For this review, take the finished solid that the model builds, in its own axes (mm). Round coordinates to 2 decimals unless told otherwise and drop trailing zeros. Write each loop counter-clockwise with the first axis right and the second up, starting at its lowest first coordinate (ties: lowest second). Pieces come first, ordered by that corner, then holes. Notation, with made-up numbers: (74.25, 36.25) - (106.25, 36.25) arc R24 ccw to (106.25, 51.25) - close; hole circle Ø4 at (9.25, -20). An arc over 180 degrees is marked (long way). Answer in a Markdown table with one row per item. Add a question column.
from build123d import *

# Parameters (mm, degrees)
SKETCH1_R           = 3.175
BOSS_EXTRUDE1_DEPTH = 3.175


with BuildPart() as part:
    # Sketch1 → Boss-Extrude1 (new body)
    with BuildSketch(Plane.XY):
        with BuildLine():
            Line((0, 38.1), (-25.4, 38.1))
            Line((-25.4, 38.1), (-25.4, 12.7))
            Line((-25.4, 12.7), (0, 12.7))
            Line((0, 12.7), (0, 9.525))
            ThreePointArc((0, 9.525), (12.7, -3.175), (25.4, 9.525))
            Line((25.4, 9.525), (25.4, 12.7))
            Line((25.4, 12.7), (50.8, 12.7))
            Line((50.8, 12.7), (50.8, 38.1))
            Line((50.8, 38.1), (25.4, 38.1))
            Line((25.4, 38.1), (25.4, 41.275))
            ThreePointArc((25.4, 41.275), (12.7, 53.975), (0, 41.275))
            Line((0, 41.275), (0, 38.1))
        make_face()
        with Locations((12.7, 44.45)):
            Circle(SKETCH1_R, mode=Mode.SUBTRACT)
        with Locations((12.7, 6.35)):
            Circle(SKETCH1_R, mode=Mode.SUBTRACT)
        with Locations((12.7, 25.4)):
            Circle(SKETCH1_R, mode=Mode.SUBTRACT)
        with Locations((38.1, 25.4)):
            Circle(SKETCH1_R, mode=Mode.SUBTRACT)
        with Locations((-12.7, 25.4)):
            Circle(SKETCH1_R, mode=Mode.SUBTRACT)
    extrude(amount=BOSS_EXTRUDE1_DEPTH)


solid = part.part
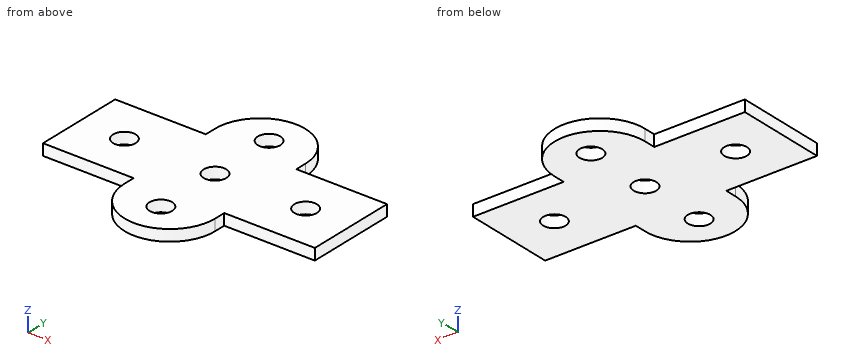
Q1. To check wall thickness, follow probe 1 along Y at (x, z) = (38.1, 1.1) (3 decimals); probe 2 along X at (y, z) = (23, 2.2); probe 3 along Y at (x, z) = (34, 2.6). State the ranges of each line that lie inside material, in increasing order.
Q2. Add section D-D on y = 6.35. State the section outline as (x, z) points (3 decimals).
Q3. Add section A-A on x = 38.1. State the section outline as (y, z) points (3 decimals).
Q4. Insertion check: pin 1 Ø1.6 at (x, z) = (-13.5, 2) entering from +Y; pin 2 Ø1.6 at (y, z) = (40, 1.5) entering from +X; pin 3 Ø8.5 at (x, y) = (38.1, 25.4) entering from -Z; pin 4 Ø1 at (x, z) = (32, 1.5) entering from -Y. Each pin has a flat end and moves straight along its axis. Give the tip position at first contact, or say it passes through.
Q5. Add section B-B on y = 25.4. State the section outline as (x, z) points (3 decimals), then the cut area to 3 significant figures.
Q6. Add section C-C on z = 1. State the section outline as (x, y) points (3 decimals), then the cut area to 3 significant figures.
Answer sheet:
| question | item | result |
|---|---|---|
| 1 | probe 1 | y = 12.7 to 22.225, 28.575 to 38.1 |
| 1 | probe 2 | x = -25.4 to -14.78, -10.62 to 10.62, 14.78 to 36.02, 40.18 to 50.8 |
| 1 | probe 3 | y = 12.7 to 38.1 |
| 2 | outline | (0.403, 0) - (9.525, 0) - (9.525, 3.175) - (0.403, 3.175) - close; (15.875, 0) - (24.997, 0) - (24.997, 3.175) - (15.875, 3.175) - close |
| 3 | outline | (12.7, 0) - (22.225, 0) - (22.225, 3.175) - (12.7, 3.175) - close; (28.575, 0) - (38.1, 0) - (38.1, 3.175) - (28.575, 3.175) - close |
| 4 | pin 1 | stops at y = 38.1 |
| 4 | pin 2 | stops at x = 25.4 |
| 4 | pin 3 | stops at z = 0 |
| 4 | pin 4 | stops at y = 12.7 |
| 5 | outline | (-25.4, 0) - (-15.875, 0) - (-15.875, 3.175) - (-25.4, 3.175) - close; (-9.525, 0) - (9.525, 0) - (9.525, 3.175) - (-9.525, 3.175) - close; (15.875, 0) - (34.925, 0) - (34.925, 3.175) - (15.875, 3.175) - close; (41.275, 0) - (50.8, 0) - (50.8, 3.175) - (41.275, 3.175) - close |
| 5 | area | 181 mm² |
| 6 | outline | (-25.4, 12.7) - (0, 12.7) - (0, 9.525) arc R12.7 ccw to (25.4, 9.525) - (25.4, 12.7) - (50.8, 12.7) - (50.8, 38.1) - (25.4, 38.1) - (25.4, 41.275) arc R12.7 ccw to (0, 41.275) - (0, 38.1) - (-25.4, 38.1) - close; hole circle Ø6.35 at (-12.7, 25.4); hole circle Ø6.35 at (12.7, 6.35); hole circle Ø6.35 at (12.7, 25.4); hole circle Ø6.35 at (12.7, 44.45); hole circle Ø6.35 at (38.1, 25.4) |
| 6 | area | 2,450 mm² |
